Job drawing, mm, ordinate dimensions from the low corner. One solid piece. Give positions to 0.01 mm unless a question says otherwise; leave off trailing zeros. Order: outer loops, then holes, each group sorted by start corner. A loop starts at its lowest first (then second) coordinate and runs counter-clockwise, first axis right, second up. Notation, with made-up numbers: (-33.5, 28.5) - (-27.5, 28.5) arc R25 cw to (-27.5, 53.5) - close; hole circle Ø6 at (-19.5, 40). An arc over 180 degrees is marked (long way). Write each question's results on one line, items separated by ' | '. Start each with the question number.
1) Drop flat-ended pins along their axis: pin 1 Ø2 at (y, z) = (5.5, 7.5) entering from +X; pin 2 Ø2.5 at (x, y) = (20, 35) entering from +Z; pin 3 Ø6 at (x, z) = (15, 2.5) entering from -Y; pin 4 Ø6 at (x, z) = (34.5, 8) entering from -Y. Give the stop position or say it passes through.
2) Two-plate mould, pull along X, no slides. Class the marked faces 1, 2 and 3: +X half, -X half, draft (parallel to the pull), parting line (faces both ways), or undercut.
3) Cut at C-C on z = 9.25. List the corners of the cut face in (x, y) (1 decimal), plus the area to 3 significant figures.
4) Drill centre lines: line 1 along Y through (x, z) = (20, 2); line 2 along X through (y, z) = (20.5, 7.75); line 3 along Y through (x, z) = (19, 4). Where is each one in solid material? Low to high. Write a range as from..to.
5) Cut at D-D on x = 35. List the corners of the cut face in (y, z), plus the area to 3 significant figures.
6) Cut at A-A on y = 20. List the corners of the cut face in (x, z), plus the area to 4 significant figures.
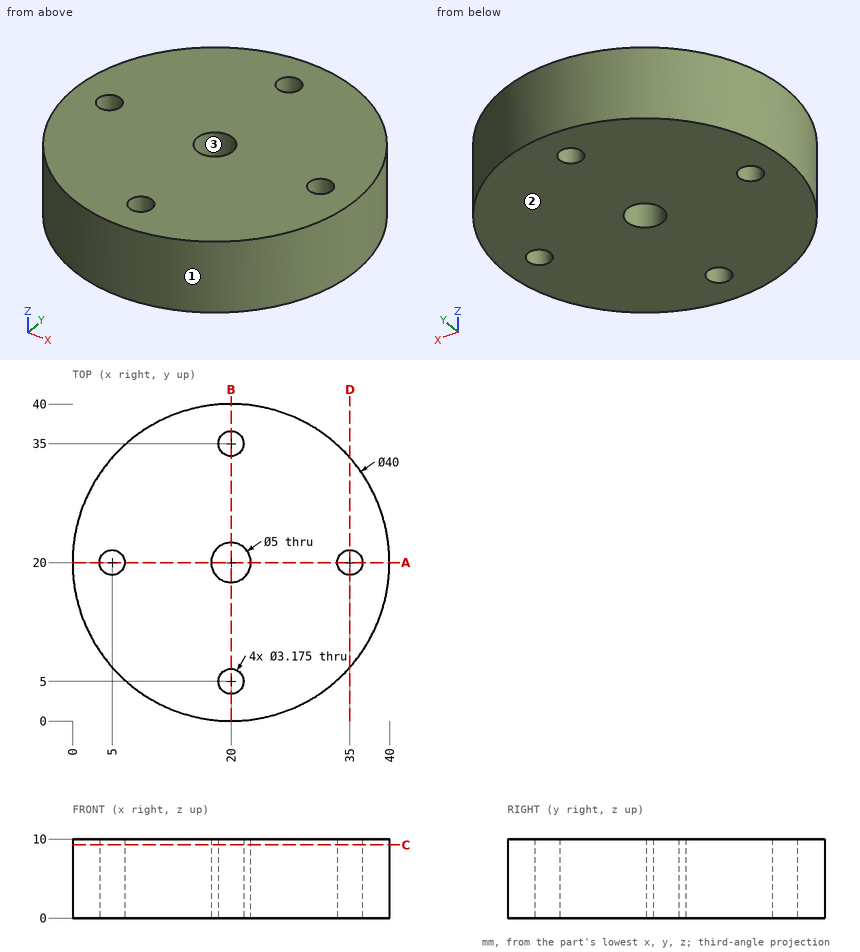
Results:
1) pin 1: x = 34.76 | pin 2: through | pin 3: y = 0.1 | pin 4: y = 3.64
2) face 1: parting line | face 2: draft | face 3: undercut
3) outline: circle Ø40 at (20, 20); hole circle Ø3.2 at (5, 20); hole circle Ø5 at (20, 20); hole circle Ø3.2 at (20, 5); hole circle Ø3.2 at (20, 35); hole circle Ø3.2 at (35, 20) | area: 1,210 mm^2
4) line 1: 0..3.41, 6.59..17.5, 22.5..33.41, 36.59..40 | line 2: 0.01..3.49, 6.51..17.55, 22.45..33.49, 36.51..39.99 | line 3: 0.03..3.77, 6.23..17.71, 22.29..33.77, 36.23..39.97
5) outline: (6.77, 0) - (18.41, 0) - (18.41, 10) - (6.77, 10) - close; (21.59, 0) - (33.23, 0) - (33.23, 10) - (21.59, 10) - close | area: 233 mm^2
6) outline: (0, 0) - (3.41, 0) - (3.41, 10) - (0, 10) - close; (6.59, 0) - (17.5, 0) - (17.5, 10) - (6.59, 10) - close; (22.5, 0) - (33.41, 0) - (33.41, 10) - (22.5, 10) - close; (36.59, 0) - (40, 0) - (40, 10) - (36.59, 10) - close | area: 286.5 mm^2
